Check sheet for the modelled part. Datum: model origin and axes. Units: mm. A direction names the side the tool comes from. Give positions to 0.01 mm unless a question says otherwise; leave off trailing zeros. Loops run counter-clockwise (first coordinate to the right, second up) from the corner with the lowest first, then second, coordinate; pieces in that order, holes last. Notation, with made-up numbers: (78.5, -37.5) - (84.5, -37.5) arc R26 ccw to (84.5, -3.5) - close; hole circle Ø3 at (64, 69). An arc over 180 degrees is marked (long way). Answer in a Markdown table with one row per item. Add a question column.
(1) Sectioned sample at A-A on y = 1.5. Enter the section's corners in (x, z), then the cut area to 3 significant figures.
(2) Thickness scan on L1, parallel to Y at x = -18, z = 23.5; L2, parallel to X at y = -17.6, z = 18.75. Record the ranges inside material, lowest first.
(3) Sectioned sample at B-B on x = 12. Enter the section's corners in (y, z).
(4) Sectioned sample at C-C on z = 27. Enter the section's corners in (x, y), then the cut area to 3 significant figures.
(5) Set-up check for faces 1 (the face through (18, -15, 25)), 2 (the face through (-0.07, 17.97, 13.5)), 3 (the face through (-17.34, -18.42, 4.06)): record each of +Z, -Z, +X, -X, +Y, -Y from which the full face is reachable in a straight line by a thin tool's end or side.
(6) Draft check along Y on faces 4 (the face through (2, 16, 15)), 5 (the face through (5.394, -18.359, 20.186)), 6 (the face through (-16.4, -1.4, 30)). Enter one of: released by +Y, released by -Y, zero draft, split by the parting line, or undercut.
(7) Go/stop test with flat-tipped pins: P1, Ø1.8, axis at x = 0, z = 15, coming from the +Y side; P2, Ø1.3, axis at x = 18, y = 18, coming from the -Z side; P3, Ø1.3, axis at x = -18, y = 18, coming from the +Z side. Record where each tip stops, or that it passes through.
(8) Sectioned sample at D-D on y = -10. Enter the section's corners in (x, z).
Autodesk Inventor part; units mm, degrees
ref_plane "Arbeitsebene1" through (0, 0, 15) normal (0, 0, 1) x (1, 0, 0)
ref_plane "YZ Plane" through (0, 0, 0) normal (1, 0, 0) x (0, 1, 0)
ref_plane "XZ Plane" through (0, 0, 0) normal (0, 1, 0) x (-1, 0, 0)
sketch "Skizze1" plane through (0, 0, 0) normal (0, 0, 1) x (1, 0, 0)
  line L0 (-20, 20) -> (20, 20)
  line L1 (20, 20) -> (20, -20)
  line L2 (20, -20) -> (-20, -20)
  line L3 (-20, -20) -> (-20, 20)
  line L4 (-28, 0) -> (28, 0)
  line L5 (0, -28) -> (0, 28)
  line L6 (16, 16) -> (-16, 16)
  line L7 (-16, 16) -> (-16, -16)
  line L8 (-16, -16) -> (16, -16)
  line L9 (16, -16) -> (16, 16)
  point P0 (0, 0)
  dimension "d0" = 40
  dimension "d1" = 4
extrude "Extrusion1" add sketch "Skizze1" along normal blind 30 contours L0 L5 L6 L7 L4 L3 | L0 L1 L4 L9 L6 L5 | L4 L7 L8 L5 L2 L3 | L1 L2 L5 L8 L9 L4
sketch "Skizze2" plane through (20, -20, 0) normal (1, 0, 0) x (0, 0, -1)
  line L0 (-30, 40) -> (-30, 0)
  line L1 (0, 0) -> (-30, 0)
  line L2 (0, 40) -> (-30, 40)
  line L3 (0, -8) -> (0, 48)
  line L4 (6, 20) -> (-36, 20)
  line L5 (-30, 36) -> (-28, 36)
  line L6 (-23, 31) -> (-23, 9)
  line L7 (-28, 4) -> (-30, 4)
  line L8 (-30, 4) -> (-30, 36)
  line L9 (0, 36) -> (-2, 36)
  line L10 (-7, 31) -> (-7, 9)
  line L11 (-2, 4) -> (0, 4)
  line L12 (0, 4) -> (0, 36)
  line L13 (-15, 40) -> (-15, 0)
  line L14 (0, 4) -> (-30, 4)
  arc A0 (-23, 31) -> (-28, 36) centre (-28, 31) ccw
  arc A1 (-28, 4) -> (-23, 9) centre (-28, 9) ccw
  arc A2 (-7, 9) -> (-2, 4) centre (-2, 9) ccw
  arc A3 (-2, 36) -> (-7, 31) centre (-2, 31) ccw
  point P0 (0, 20)
  dimension "d5" = 16
  dimension "d6" = 5
extrude "Extrusion2" cut sketch "Skizze2" against normal up to surface (4 mm away) contours L5 A0 L6 L4 L0 | L4 L6 A1 L7 L0 | L3 L4 L10 A3 L9 | L4 L3 L11 A2 L10
sketch "Skizze3" plane through (-20, -20, 0) normal (0, -1, 0) x (1, 0, 0)
  line L0 (40, 30) -> (0, 30)
  line L1 (0, 0) -> (0, 30)
  line L2 (40, 0) -> (40, 30)
  line L3 (20, 30) -> (20, 0)
  line L4 (0, 15) -> (40, 15)
  circle A0 centre (20, 15) radius 7.5
  line L5 (13.5048, 18.75) -> (20, 15)
  line L6 (20, 15) -> (26.4952, 18.75)
  point P0 (20, 7.5)
  dimension "d9" = 15
  dimension "d10" = 60
  dimension "d11" = 60
hole "Bohrung1" at (0, -20, 7.5) at (-6.4952, -20, 18.75) at (6.4952, -20, 18.75) direction (0, 1, 0) diameter 3.4 end up to surface countersink diameter 6.9 countersink angle 90
sketch "Skizze4" plane through (20, -20, 0) normal (1, 0, 0) x (0, 0, -1)
  circle A0 centre (-15, 29) radius 2.25
  circle A1 centre (-15, 11) radius 2.25
  point P0 (0, 20)
hole "Bohrung2" at (20, 9, 15) at (20, -9, 15) direction (-1, 0, 0) diameter 3.242 end up to surface
sketch "Skizze5" plane through (0, 0, 30) normal (0, 0, 1) x (1, 0, 0)
  line L0 (-20, 20) -> (20, 20)
  line L1 (-20, -20) -> (-20, 20)
  line L2 (20, -20) -> (-20, -20)
  line L3 (20, -16) -> (20, -20)
  line L4 (-18, 18) -> (18, 18)
  line L5 (18, 18) -> (18, -18)
  line L6 (18, -18) -> (-18, -18)
  line L7 (-18, -18) -> (-18, 18)
  point P0 (0, 0)
  dimension "d29" = 2
  dimension "d30" = 2
  dimension "d31" = 2
  dimension "d32" = 2
hole "Bohrung3" at (-18, 18, 30) at (18, 18, 30) at (18, -18, 30) at (-18, -18, 30) direction (0, 0, -1) diameter 1.567 depth 8 tip angle 118
ref_plane "Arbeitsebene1" through (0, 0, 15) normal (0, 0, 1) x (1, 0, 0)
mirror "Spiegeln1" about plane through (0, 0, 15) normal (0, 0, 1) of "Bohrung3"
sketch "Skizze6" plane through (-20, 20, 0) normal (0, 1, 0) x (1, 0, 0)
  line L0 (0, -30) -> (40, -30)
  line L1 (40, 0) -> (40, -30)
  line L2 (0, 0) -> (0, -30)
  line L3 (0, -15) -> (40, -15)
  line L4 (20, 0) -> (20, -30)
  point P0 (20, -15)
hole "Bohrung4" at (0, 20, 15) direction (0, -1, 0) diameter 3 depth 8 tip angle 118
properties part number "13_0204_015"
Reply:
| question | item | result |
|---|---|---|
| 1 | outline | (-20, 0) - (-16, 0) - (-16, 30) - (-20, 30) - close; (16, 7) - (20, 7) - (20, 23) - (16, 23) - close |
| 1 | area | 184 mm^2 |
| 2 | L1 | -20 to -18.78, -17.22 to 17.22, 18.78 to 20 |
| 2 | L2 | -20 to -8.2, -4.8 to 4.8, 8.2 to 20 |
| 3 | outline | (-20, 0) - (-16, 0) - (-16, 30) - (-20, 30) - close; (16, 0) - (20, 0) - (20, 30) - (16, 30) - close |
| 4 | outline | (-20, -20) - (20, -20) - (20, -15.9) - (16, -15.9) - (16, -16) - (-16, -16) - (-16, 16) - (16, 16) - (16, 15.9) - (20, 15.9) - (20, 20) - (-20, 20) - close; hole circle Ø1.57 at (-18, -18); hole circle Ø1.57 at (-18, 18); hole circle Ø1.57 at (18, -18); hole circle Ø1.57 at (18, 18) |
| 4 | area | 441 mm^2 |
| 5 | face 1 | +Z, +X |
| 5 | face 2 | +Y |
| 5 | face 3 | -Z |
| 6 | face 4 | undercut |
| 6 | face 5 | released by -Y |
| 6 | face 6 | zero draft |
| 7 | P1 | y = -16 |
| 7 | P2 | z = 8.08 |
| 7 | P3 | z = 21.92 |
| 8 | outline | (-20, 0) - (-16, 0) - (-16, 30) - (-20, 30) - close; (16, 7) - (20, 7) - (20, 13.72) - (16, 13.72) - close; (16, 16.28) - (20, 16.28) - (20, 23) - (16, 23) - close |
